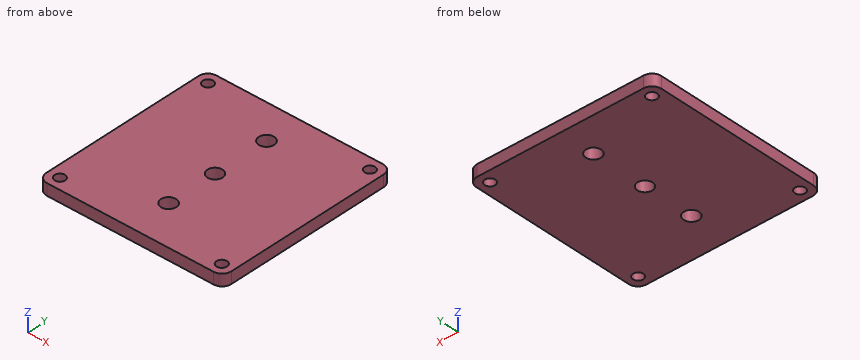
```python
from build123d import *

# Parameters (mm, degrees)
BOSS_EXTRU_1_DEPTH      = 5
D_GAGEMENT_M41_D        = 4.5
ESQUISSE4_R             = 3.25
ENL_V_MAT_EXTRU_1_DEPTH = 57.789083458
D_GAGEMENT_M61_D        = 6.6


with BuildPart() as part:
    # Esquisse1 → Boss.-Extru.1 (new body)
    with BuildSketch(Plane.XY):
        with BuildLine():
            Line((-36, -40), (36, -40))
            ThreePointArc((36, -40), (38.828427125, -38.828427125), (40, -36))
            Line((40, -36), (40, 36))
            ThreePointArc((40, 36), (38.828427125, 38.828427125), (36, 40))
            Line((36, 40), (-36, 40))
            ThreePointArc((-36, 40), (-38.828427125, 38.828427125), (-40, 36))
            Line((-40, 36), (-40, -36))
            ThreePointArc((-40, -36), (-38.828427125, -38.828427125), (-36, -40))
        make_face()
    extrude(amount=BOSS_EXTRU_1_DEPTH)

    # Dégagement M41 (through all)
    with Locations(Plane.XY.offset(5)):
        with Locations((-35.007622699, 34.962380164), (34.968353645, 34.962380164), (34.968353645, -35.023881333), (-35.007622699, -35.023881333)):
            Hole(D_GAGEMENT_M41_D / 2)

    # Esquisse4 → Enlèv. mat.-Extru.1 (cut, through all)
    with BuildSketch(Plane(origin=(0, 0, 0), x_dir=(-1, 0, 0), z_dir=(0, 0, -1))):
        Circle(ESQUISSE4_R)
    extrude(amount=-ENL_V_MAT_EXTRU_1_DEPTH, mode=Mode.SUBTRACT)

    # Dégagement M61 (through all)
    with Locations(Plane(origin=(0, 0, 0), x_dir=(-1, 0, 0), z_dir=(0, 0, -1))):
        with Locations((0, -21.916448078), (0, 24.346376155)):
            Hole(D_GAGEMENT_M61_D / 2)


solid = part.part
```
Geometry check sheet. Reference: the model listing, model coordinates, mm. Give positions to 0.01 mm unless a question says otherwise; leave off trailing zeros. Order: outer loops, then holes, each group sorted by start corner. A loop starts at its lowest first (then second) coordinate and runs counter-clockwise, first axis right, second up. Notation, with made-up numbers: (13.5, -7.5) - (26.5, -7.5) arc R17 cw to (26.5, 25.5) - close; hole circle Ø3 at (61, 42.5). An arc over 180 degrees is marked (long way). Write item = value, one per line. Start each with the question number.
1) Section check A-A (x = 0). Enter the section's corners in (y, z).
2) Scan lines: L1, parallel to Y at x = 0, z = 2.1; L2, parallel to X at y = -22, z = 3.65; L3, parallel to Y at x = -1.5, z = 3.4. Record each from-to range of solid material in increasing order.
3) Section check C-C (z = 3.8). Enter the section's corners in (x, y).
4) Section check B-B (y = 0). Enter the section's corners in (x, z), then the cut area to 4 significant figures.
5) Gauge pin test, flat end, axial feed: pin 1 Ø4 at (x, y) = (-35.01, 34.96) entering from +Z (3 decimals). Record the tip position at first contact, or that the pin passes through.
Geometry check:
q1.outline = (-40, 0) - (-25.22, 0) - (-25.22, 5) - (-40, 5) - close; (-18.62, 0) - (-3.25, 0) - (-3.25, 5) - (-18.62, 5) - close; (3.25, 0) - (21.05, 0) - (21.05, 5) - (3.25, 5) - close; (27.65, 0) - (40, 0) - (40, 5) - (27.65, 5) - close
q2.L1 = -40 to -25.22, -18.62 to -3.25, 3.25 to 21.05, 27.65 to 40
q2.L2 = -40 to -3.3, 3.3 to 40
q2.L3 = -40 to -24.86, -18.98 to -2.88, 2.88 to 21.41, 27.29 to 40
q3.outline = (-40, -36) arc R4 ccw to (-36, -40) - (36, -40) arc R4 ccw to (40, -36) - (40, 36) arc R4 ccw to (36, 40) - (-36, 40) arc R4 ccw to (-40, 36) - close; hole circle Ø4.5 at (-35.01, -35.02); hole circle Ø4.5 at (-35.01, 34.96); hole circle Ø6.6 at (0, -21.92); hole circle Ø6.6 at (0, 24.35); hole circle Ø6.5 at (0, 0); hole circle Ø4.5 at (34.97, -35.02); hole circle Ø4.5 at (34.97, 34.96)
q4.outline = (-40, 0) - (-3.25, 0) - (-3.25, 5) - (-40, 5) - close; (3.25, 0) - (40, 0) - (40, 5) - (3.25, 5) - close
q4.area = 367.5 mm2
q5.pin_1 = through
